from build123d import *

# Parameters (mm, degrees)
SKETCH_R      = 10
PAD_DEPTH     = 110
SKETCH001_R   = 10
SKETCH001_R_2 = 3.25
POCKET_DEPTH  = 7
SKETCH002_R   = 50
PAD001_DEPTH  = 5
FILLET_R      = 2
FILLET001_R   = 4
FILLET002_R   = 1
FILLET003_R   = 4


with BuildPart() as part:
    # Sketch → Pad (new body)
    with BuildSketch(Plane.XY):
        Circle(SKETCH_R)
    extrude(amount=PAD_DEPTH)

    # Sketch001 (on Face3 of Pad) → Pocket (cut)
    with BuildSketch(Plane.XY.offset(110)):
        Circle(SKETCH001_R)
        Circle(SKETCH001_R_2, mode=Mode.SUBTRACT)
    extrude(amount=-POCKET_DEPTH, mode=Mode.SUBTRACT)

    # Sketch002 (on Face2 of Pocket) → Pad001 (join)
    with BuildSketch(Plane(origin=(0, 0, 0), x_dir=(1, 0, 0), z_dir=(0, 0, -1))):
        Circle(SKETCH002_R)
    extrude(amount=PAD001_DEPTH)

    # Fillet
    fillet_edges = [part.edges().sort_by_distance(p)[0] for p in [
        (-50, 0, -5),
        (-50, 0, 0),
    ]]
    fillet(fillet_edges, radius=FILLET_R)

    # Fillet001
    fillet001_edges = [part.edges().sort_by_distance(p)[0] for p in [
        (-10, 0, 103),
    ]]
    fillet(fillet001_edges, radius=FILLET001_R)

    # Fillet002
    fillet002_edges = [part.edges().sort_by_distance(p)[0] for p in [
        (-3.25, 0, 110),
    ]]
    fillet(fillet002_edges, radius=FILLET002_R)

    # Fillet003
    fillet003_edges = [part.edges().sort_by_distance(p)[0] for p in [
        (-10, 0, 0),
    ]]
    fillet(fillet003_edges, radius=FILLET003_R)


solid = part.part
Could you check a few things on this model? Use its own coordinates, in mm. A direction names the side the tool comes from. Coordinates: 2 decimals unless noted, no trailing zeros. Loops run counter-clockwise (first coordinate to the right, second up) from the corner with the lowest first, then second, coordinate; pieces in that order, holes last.
1. I need wall thicknesses on L1, parallel to Z at x = -26.5, y = -3; L2, parallel to Y at x = -5.5, z = 17.5; L3, parallel to X at y = -3, z = 32.5. Which ranges of each line are inside material? Lowest first, please.
2. Imagine slicing it at A-A (x = 0). Please give me the cut outline in (y, z).
3. Imagine slicing it at C-C (z = 91.5). Please give me the cut outline in (x, y), and give its area (3 significant figures).
4. For faces 1 (the face through (3, -3, 103)), 2 (the face through (47.69, -15.02, -2.49)), which set-ups out of +Z, -Z, +X, -X, +Y, -Y let a thin tool reach every point of the face, with its end or its side?
5. For P1, Ø13, axis at x = -1.5, y = -2, coming from the +Z side; P2, Ø1, axis at x = 32, y = 2.5, coming from the +Z side; P3, Ø10, axis at y = -14, z = 89.5, coming from the -X side; P4, Ø12, axis at x = 6.5, z = 13.5, coming from the +Y side, each with a flat end and sliding along its axis, tell me the tip position at first contact or that it passes through.
Computed values:
1. L1: z = -5 to 0
1. L2: y = -8.35 to 8.35
1. L3: x = -9.54 to 9.54
2. outline: (-50, -3) arc R2 ccw to (-48, -5) - (48, -5) arc R2 ccw to (50, -3) - (50, -2) arc R2 ccw to (48, 0) - (14, 0) arc R4 cw to (10, 4) - (10, 99) arc R4 ccw to (6, 103) - (3.25, 103) - (3.25, 109) arc R1 ccw to (2.25, 110) - (-2.25, 110) arc R1 ccw to (-3.25, 109) - (-3.25, 103) - (-6, 103) arc R4 ccw to (-10, 99) - (-10, 4) arc R4 cw to (-14, 0) - (-48, 0) arc R2 ccw to (-50, -2) - close
3. outline: circle Ø20 at (0, 0)
3. area: 314 mm2
4. face 1: +Z
4. face 2: +Z, -Z
5. P1: stops at z = 110
5. P2: stops at z = 0
5. P3: stops at x = -4.36
5. P4: stops at y = 9.99
